Source: CAD feature listing. Evaluate the final solid. Frame: model axes, mm. Round coordinates to 2 decimals unless told otherwise and drop trailing zeros. Order: outer loops, then holes, each group sorted by start corner. A loop starts at its lowest first (then second) coordinate and runs counter-clockwise, first axis right, second up.
```python
from build123d import *

# Parameters (mm, degrees)
BOSS_EXTRUDE1_DEPTH      = 15
BOSS_EXTRUDE1_DEPTH_BACK = 3
SHELL1_T                 = -1
SKETCH2_R                = 3
SKETCH2_R_2              = 1.5
BOSS_EXTRUDE2_DEPTH      = 6
SKETCH4_W                = 9.424257845
SKETCH4_H                = 10.522525497
CUT_EXTRUDE1_DEPTH       = 10


with BuildPart() as part:
    # Sketch1 → Boss-Extrude1 (new, two sides: drawn at the far end of the back side and taken through both)
    with BuildSketch(Plane(origin=(0, 0, 0), x_dir=(1, 0, 0), z_dir=(0, 1, 0)).offset(-BOSS_EXTRUDE1_DEPTH_BACK)):
        with BuildLine():
            Line((-68, -50), (68, -50))
            ThreePointArc((68, -50), (69.414213562, -49.414213562), (70, -48))
            Line((70, -48), (70, 48))
            ThreePointArc((70, 48), (69.414213562, 49.414213562), (68, 50))
            Line((68, 50), (-68, 50))
            ThreePointArc((-68, 50), (-69.414213562, 49.414213562), (-70, 48))
            Line((-70, 48), (-70, -48))
            ThreePointArc((-70, -48), (-69.414213562, -49.414213562), (-68, -50))
        make_face()
    extrude(amount=BOSS_EXTRUDE1_DEPTH + BOSS_EXTRUDE1_DEPTH_BACK)

    # Shell1
    shell1_openings = [part.faces().sort_by_distance(p)[0] for p in [
        (0, 15, 0),
    ]]
    offset(amount=SHELL1_T, openings=shell1_openings, kind=Kind.INTERSECTION)

    # Sketch2 → Boss-Extrude2 (add)
    # profile 1 of 4: a face of its own
    with BuildSketch(Plane(origin=(0, -2, 0), x_dir=(1, 0, 0), z_dir=(0, 1, 0))):
        with Locations(Location((-57.5, 35.380535612, 0), (0, 0, 270))):
            Circle(SKETCH2_R)
        with Locations(Location((-57.5, 35.380535612, 0), (0, 0, 270))):
            Circle(SKETCH2_R_2, mode=Mode.SUBTRACT)
    # profile 2 of 4: a face of its own
    with BuildSketch(Plane(origin=(0, -2, 0), x_dir=(1, 0, 0), z_dir=(0, 1, 0))):
        with Locations(Location((-57.5, 12.968164447, 0), (0, 0, 270))):
            Circle(SKETCH2_R)
        with Locations(Location((-57.5, 12.968164447, 0), (0, 0, 270))):
            Circle(SKETCH2_R_2, mode=Mode.SUBTRACT)
    # profile 3 of 4: a face of its own
    with BuildSketch(Plane(origin=(0, -2, 0), x_dir=(1, 0, 0), z_dir=(0, 1, 0))):
        with Locations(Location((57.5, 12.968164447, 0), (0, 0, 90))):
            Circle(SKETCH2_R)
        with Locations(Location((57.5, 12.968164447, 0), (0, 0, 90))):
            Circle(SKETCH2_R_2, mode=Mode.SUBTRACT)
    # profile 4 of 4: a face of its own
    with BuildSketch(Plane(origin=(0, -2, 0), x_dir=(1, 0, 0), z_dir=(0, 1, 0))):
        with Locations(Location((57.5, 35.380535612, 0), (0, 0, 90))):
            Circle(SKETCH2_R)
        with Locations(Location((57.5, 35.380535612, 0), (0, 0, 90))):
            Circle(SKETCH2_R_2, mode=Mode.SUBTRACT)
    extrude(amount=BOSS_EXTRUDE2_DEPTH)

    # Sketch4 → Cut-Extrude1 (cut)
    with BuildSketch(Plane.XY.offset(50)):
        with Locations((-37.455086441, 10.521410827)):
            Rectangle(SKETCH4_W, SKETCH4_H)
    extrude(amount=-CUT_EXTRUDE1_DEPTH, mode=Mode.SUBTRACT)


solid = part.part
```
1. Section A-A on y = 1. State how many separate pieces and enclosed holes the cut face has, plus the area to 3 significant figures.
2. Section C-C on z = 12. Return loops of the section in (x, y), plus the area to 3 significant figures.
3. Pull-direction query (Z, two-part tool) for faces 1 (the face through (-1, 6, 50)), 2 (the face through (70, 6, 1)), 3 (the face through (56.235, 0.958, -13.775)); classes: released by +Z, released by -Z, zero draft, split by the parting line, or undercut.
4. First-contact query: pin 1 (3.5 mm diameter, centred on x = 58, z = -35.5, fed in from +Y); pin 2 (1.8 mm diameter, centred on x = -57.5, z = -35, fed in from +Y); pin 3 (1.1 mm diameter, centred on x = -35.5, z = 49.5, fed in from +Y). Flat tips, straight axial feed; report the tip coordinate or a pass-through.
5. Section D-D on x = 39. Return loops of the section in (y, z), plus the area to 3 significant figures.
6. Line query: line 1 along Z through (x, y) = (57.5, 0.4); line 2 along X through (y, z) = (7.5, 30.5); line 3 along Z through (x, y) = (7.5, 12.25). Output: solid intervals per line, ascending.
7. Section B-B on x = 57.5. Return loops of the section in (y, z), plus the area to 3 significant figures.
Result:
1. separate pieces: 5
1. enclosed holes: 5
1. area: 558 mm2
2. outline: (-70, -3) - (70, -3) - (70, 15) - (69, 15) - (69, -2) - (-69, -2) - (-69, 15) - (-70, 15) - close
2. area: 174 mm2
3. face 1: released by +Z
3. face 2: zero draft
3. face 3: undercut
4. pin 1: stops at y = 4
4. pin 2: stops at y = -2
4. pin 3: stops at y = 5.26
5. outline: (-3, -50) - (15, -50) - (15, -49) - (-2, -49) - (-2, 49) - (15, 49) - (15, 50) - (-3, 50) - close
5. area: 134 mm2
6. line 1: z = -50 to -49, -38.38 to -36.88, -33.88 to -32.38, -15.97 to -14.47, -11.47 to -9.97, 49 to 50
6. line 2: x = -70 to -69, 69 to 70
6. line 3: z = -50 to -49, 49 to 50
7. outline: (-3, -50) - (15, -50) - (15, -49) - (-2, -49) - (-2, -38.38) - (4, -38.38) - (4, -36.88) - (-2, -36.88) - (-2, -33.88) - (4, -33.88) - (4, -32.38) - (-2, -32.38) - (-2, -15.97) - (4, -15.97) - (4, -14.47) - (-2, -14.47) - (-2, -11.47) - (4, -11.47) - (4, -9.97) - (-2, -9.97) - (-2, 49) - (15, 49) - (15, 50) - (-3, 50) - close
7. area: 170 mm2
